Autodesk Inventor part; units mm, degrees
ref_plane "YZ Plane" through (0, 0, 0) normal (1, 0, 0) x (0, 1, 0)
ref_plane "XZ Plane" through (0, 0, 0) normal (0, 1, 0) x (-1, 0, 0)
ref_plane "XY Plane" through (0, 0, 0) normal (0, 0, 1) x (1, 0, 0)
sketch "Эскиз1" plane through (0, 0, 0) normal (0, 0, 1) x (1, 0, 0)
  circle A0 centre (0, 0) radius 15
  circle A1 centre (0, 6.5) radius 1.35 construction
  circle A2 centre (-5.6292, -3.25) radius 1.35 construction
  circle A3 centre (5.6292, -3.25) radius 1.35 construction
  circle A4 centre (0, 0) radius 1.1
  dimension "d0" = 30
  dimension "d1" = 2.7
  dimension "d2" = 6.5
  dimension "d5" = 360
  dimension "d21" = 2.2
extrude "Выдавливание1" add sketch "Эскиз1" along normal blind 6 contours A0 | A4
fillet "Сопряжение1" radius 2 1 edges at (-15, 0, 6)
sketch "Эскиз4" plane through (0, 0, 6) normal (0, 0, 1) x (1, 0, 0)
  circle A0 centre (0, 0) radius 2.2
  dimension "d22" = 4.4
extrude "Выдавливание4" cut sketch "Эскиз4" against normal blind 10
sketch "Эскиз5" plane through (0, 0, 0) normal (0, 0, -1) x (-1, 0, 0)
  circle A0 centre (0, 0) radius 9.15
  dimension "d28" = 18.3
extrude "Выдавливание5" cut sketch "Эскиз5" against normal blind 0.8
properties part number "крышка"
For this review, take the finished solid that the model builds, in its own axes (mm). A direction names the side the tool comes from. Round coordinates to 2 decimals unless told otherwise and drop trailing zeros. Write each loop counter-clockwise with the first axis right and the second up, starting at its lowest first coordinate (ties: lowest second). Pieces come first, ordered by that corner, then holes. Notation, with made-up numbers: (12, 75) - (24, 75) arc R14 cw to (24, 89) - close; hole circle Ø6 at (24.25, 9). An arc over 180 degrees is marked (long way). Write each question's results on one line, items separated by ' | '.
Item 1: For pin 1 (5.5 mm diameter, centred on x = -4, y = 2, fed in from -Z); pin 2 (3 mm diameter, centred on y = -11.5, z = 1, fed in from +X); pin 3 (2 mm diameter, centred on x = -9.5, z = 4.5, fed in from -Y); pin 4 (3.5 mm diameter, centred on x = 0, y = 0, fed in from -Z), all flat-tipped, find the tip position at first contact; note any pin that passes through.
Calculated:
pin 1: stops at z = 0.8 | pin 2: stops at x = 11.18 | pin 3: stops at y = -12.32 | pin 4: passes through
Item 2: Take a section at A-A on x = 0. State the section outline as (y, z) points, then the cut area to 3 significant figures.
Calculated:
outline: (-15, 0) - (-9.15, 0) - (-9.15, 0.8) - (-2.2, 0.8) - (-2.2, 6) - (-13, 6) arc R2 ccw to (-15, 4) - close; (2.2, 0.8) - (9.15, 0.8) - (9.15, 0) - (15, 0) - (15, 4) arc R2 ccw to (13, 6) - (2.2, 6) - close | area: 141 mm^2
Item 3: Draft analysis for pull direction Y (two halves, no side actions). For faces 3 (the face through (-6.9, -6.5, 0)), 4 (the face through (-2, -2, 0.8)), 5 (the face through (-14.985, -0.66, 1.972)), state which applies: pulls with the +Y half, pulls with the -Y half, needs draft (parallel to the pull), parting line crosses it, or undercut.
Calculated:
face 3: needs draft | face 4: undercut | face 5: parting line crosses it
Item 4: To check wall thickness, follow line 1 along Y through (x, z) = (0, 3.4); line 2 along Z through (x, y) = (-3.75, -5.75); line 3 along Z through (x, y) = (11.5, -6.25). State the ranges of each line that lie inside material, in increasing order. Write a range as from..to.
Calculated:
line 1: y = -15..-2.2, 2.2..15 | line 2: z = 0.8..6 | line 3: z = 0..6
Item 5: For faces 1 (the face through (-4.919, 7.715, 0.394)), 2 (the face through (3, 0, 6)), list the 3-axis set-ups (+Z, -Z, +X, -X, +Y, -Y) from which the entire face can be reached by the end or side of a thin tool; tool diameter is ignored.
Calculated:
face 1: -Z | face 2: +Z, +X, -X, +Y, -Y
Item 6: Take a section at C-C on z = 4.95. State the section outline as (x, y) points.
Calculated:
outline: circle Ø29.52 at (0, 0); hole circle Ø4.4 at (0, 0)
